Drawing for the job (mm, zero at the part's lowest x, y, z). A direction names the side the tool comes from. Round coordinates to 2 decimals unless told otherwise and drop trailing zeros. Loops run counter-clockwise (first coordinate to the right, second up) from the corner with the lowest first, then second, coordinate; pieces in that order, holes last. Notation, with made-up numbers: M 85,63 L 101,63 A24 cw 101,80 Z; hole C 31.5,24 d4. An arc over 180 degrees is marked long. Use a Markdown table: item, result. Add a question column.
Q1. Cut at B-B (x = 20.5). Give the cut face in (y, z), plus the area to 4 significant figures.
Q2. Pin check, flat tip, straight feed: pin 1 (6 mm diameter, centred on x = 39, y = 5.5, fed in from -Z). Stop position of the tip, or through.
Q3. Cut at C-C (y = 8). Give the cut face in (x, z), plus the area to 3 significant figures.
Q4. Probe line 1 (X direction, y = 15, z = 17); line 2 (Y direction, x = 29, z = 59); line 3 (Z direction, x = 51.5, y = 75). List the from-to ranges inside material, lowest first. Write a range as from..to.
Q5. Mould opens along Y. For the marked faces 3, 4, 5 and 6 say: +Y half, -Y half, draft (parallel to the pull), parting line (faces both ways), or undercut.
Q6. Cut at A-A (z = 37.5). Give the cut face in (x, y).
Q7. Tool access for the marked faces 1 and 2: list every direction of +Z, -Z, +X, -X, +Y, -Y with a clear straight run to the whole face (end or side of a thin tool).
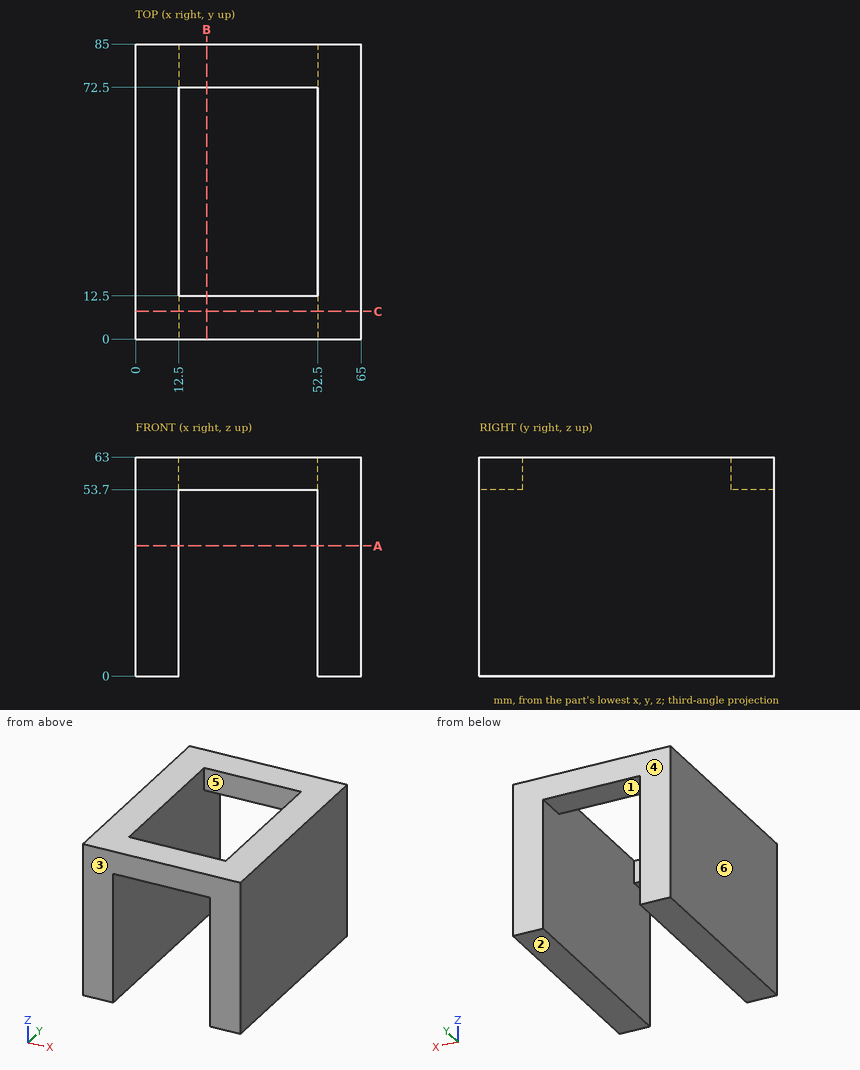
Checked values:
| question | item | result |
|---|---|---|
| 1 | outline | M 0,53.7 L 12.5,53.7 L 12.5,63 L 0,63 Z; M 72.5,53.7 L 85,53.7 L 85,63 L 72.5,63 Z |
| 1 | area | 232.5 mm^2 |
| 2 | pin 1 | stops at z = 53.7 |
| 3 | outline | M 0,0 L 12.5,0 L 12.5,53.7 L 52.5,53.7 L 52.5,0 L 65,0 L 65,63 L 0,63 Z |
| 3 | area | 1,950 mm^2 |
| 4 | line 1 | x = 0..12.5, 52.5..65 |
| 4 | line 2 | y = 0..12.5, 72.5..85 |
| 4 | line 3 | z = 53.7..63 |
| 5 | face 3 | -Y half |
| 5 | face 4 | +Y half |
| 5 | face 5 | undercut |
| 5 | face 6 | draft |
| 6 | outline | M 0,0 L 12.5,0 L 12.5,85 L 0,85 Z; M 52.5,0 L 65,0 L 65,85 L 52.5,85 Z |
| 7 | face 1 | -Z, +Y, -Y |
| 7 | face 2 | -Z, +X, -X, +Y, -Y |
